```python
from build123d import *

# Parameters (mm, degrees)
SKETCH1_R           = 1.55
BOSS_EXTRUDE1_DEPTH = 3


with BuildPart() as part:
    # Sketch1 → Boss-Extrude1 (new body)
    with BuildSketch(Plane.XY):
        with BuildLine():
            Line((46.57384356, 8.887676402), (45.062968853, 8.887676402))
            ThreePointArc((45.062968853, 8.887676402), (40.054584258, 4.478002756), (33.57384356, 2.887676402))
            Line((33.57384356, 2.887676402), (15.07384356, 2.887676402))
            Line((15.07384356, 2.887676402), (15.07384356, 0.887676439))
            Line((15.07384356, 0.887676439), (15.07384356, -1.112323636))
            Line((15.07384356, -1.112323636), (15.07384356, -9.112323598))
            Line((15.07384356, -9.112323598), (50.07384356, -9.112323598))
            Line((50.07384356, -9.112323598), (50.07384356, 8.887676402))
            Line((50.07384356, 8.887676402), (48.573843574, 8.887676402))
            Line((48.573843574, 8.887676402), (46.57384356, 8.887676402))
        make_face()
        with Locations((18.07384356, -5.112323598)):
            Circle(SKETCH1_R, mode=Mode.SUBTRACT)
        with Locations((47.07384356, -5.112323598)):
            Circle(SKETCH1_R, mode=Mode.SUBTRACT)
    extrude(amount=BOSS_EXTRUDE1_DEPTH)


solid = part.part
```
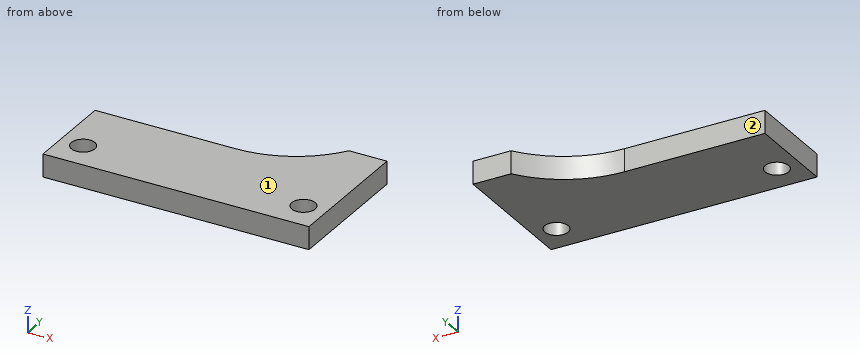
Work out the finished part from the listing and answer in its coordinate system (mm). Face numbers are marked on the shaded views. A direction names the side the tool comes from. Give positions to 0.01 mm unless a question says otherwise; leave off trailing zeros. Loops run counter-clockwise (first coordinate to the right, second up) from the corner with the lowest first, then second, coordinate; pieces in that order, holes last. Notation, with made-up numbers: (11, -29.75) - (41, -29.75) arc R22 ccw to (41, 6.25) - close; hole circle Ø3 at (4, 9.25). An arc over 180 degrees is marked (long way). Use CSV: the item, a comma, the result in double quotes. Start each with the question number.
(1) A tool of negligible diameter and unlimited length cuts with its end or side. For the marked faces 1 and 2, from which of +Z, -Z, +X, -X, +Y, -Y can it reach the whole face along a straight path? Write none if from no direction.
(2) Find section C-C, the plane y = 4.5. Determine the outline of the cut face in (x, z), plus the area to 3 significant figures.
(3) Find the intervals of material crossed by L1, parallel to X at y = -6.5, z = 1.2; L2, parallel to Y at x = 47, z = 2.5; L3, parallel to Y at x = 19, z = 1.2, in increasing order.
(4) Find section D-D, the plane x = 29. Determine the outline of the cut face in (y, z).
(5) Find section A-A, the plane z = 0.5. Determine the outline of the cut face in (x, y).
(6) Find section B-B, the plane x = 19. Determine the outline of the cut face in (y, z).
(7) Each of these flat-tipped pins is pushed along its axis until it touches: pin 1 (1.5 mm diameter, centred on x = 23.5, z = 1.5, fed in from +Y); pin 2 (1.5 mm diameter, centred on y = 5.5, z = 1.5, fed in from -X). Where does it stop, or does it pass through?
Results found:
1,face 1,"+Z, +X, -X, +Y, -Y"
1,face 2,"+Z, -Z, -X, +Y"
2,outline,"(40.1, 0) - (50.07, 0) - (50.07, 3) - (40.1, 3) - close"
2,area,"29.9 mm^2"
3,L1,"15.07 to 17.38, 18.76 to 46.38, 47.76 to 50.07"
3,L2,"-9.11 to -6.66, -3.56 to 8.89"
3,L3,"-9.11 to -6.36, -3.87 to 2.89"
4,outline,"(-9.11, 0) - (2.89, 0) - (2.89, 3) - (-9.11, 3) - close"
5,outline,"(15.07, -9.11) - (50.07, -9.11) - (50.07, 8.89) - (45.06, 8.89) arc R14 cw to (33.57, 2.89) - (15.07, 2.89) - close; hole circle Ø3.1 at (18.07, -5.11); hole circle Ø3.1 at (47.07, -5.11)"
6,outline,"(-9.11, 0) - (-6.36, 0) - (-6.36, 3) - (-9.11, 3) - close; (-3.87, 0) - (2.89, 0) - (2.89, 3) - (-3.87, 3) - close"
7,pin 1,"y = 2.89"
7,pin 2,"x = 40.55"
